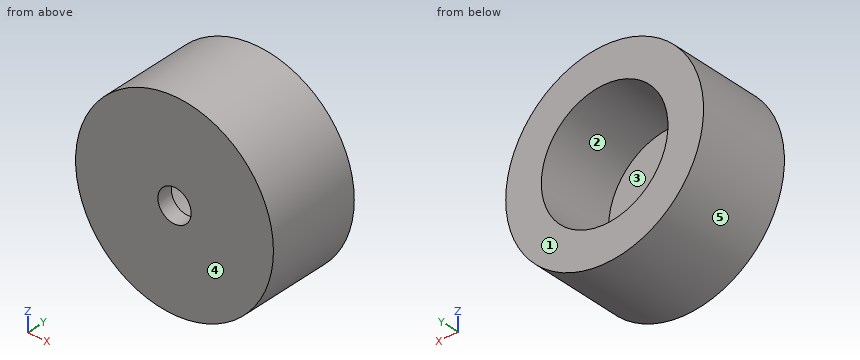
from build123d import *

# Parameters (mm, degrees)
SKETCH1_R           = 12.5
BOSS_EXTRUDE1_DEPTH = 2
SKETCH2_R           = 12.5
SKETCH2_R_2         = 8
BOSS_EXTRUDE2_DEPTH = 10
SKETCH3_R           = 2.1
CUT_EXTRUDE1_DEPTH  = 10


with BuildPart() as part:
    # Sketch1 → Boss-Extrude1 (new body)
    with BuildSketch(Plane(origin=(0, 0, 0), x_dir=(1, 0, 0), z_dir=(0, 1, 0))):
        Circle(SKETCH1_R)
    extrude(amount=BOSS_EXTRUDE1_DEPTH)

    # Sketch2 → Boss-Extrude2 (add)
    with BuildSketch(Plane(origin=(0, 2, 0), x_dir=(1, 0, 0), z_dir=(0, 1, 0))):
        Circle(SKETCH2_R)
        Circle(SKETCH2_R_2, mode=Mode.SUBTRACT)
    extrude(amount=BOSS_EXTRUDE2_DEPTH)

    # Sketch3 → Cut-Extrude1 (cut)
    with BuildSketch(Plane(origin=(0, 2, 0), x_dir=(1, 0, 0), z_dir=(0, 1, 0))):
        Circle(SKETCH3_R)
    extrude(amount=-CUT_EXTRUDE1_DEPTH, mode=Mode.SUBTRACT)


solid = part.part
Check sheet for the modelled part. Datum: model origin and axes. Units: mm. Face numbers are marked on the shaded views. A direction names the side the tool comes from. Give positions to 0.01 mm unless a question says otherwise; leave off trailing zeros. Order: outer loops, then holes, each group sorted by start corner. A loop starts at its lowest first (then second) coordinate and runs counter-clockwise, first axis right, second up. Notation, with made-up numbers: M 74.5,-39.5 L 96.5,-39.5 A35 ccw 96.5,-0.5 Z; hole C -3.75,-29.5 d2. An arc over 180 degrees is marked long. Answer as CSV lines item,"result". Start each with the question number.
Item 1: Cross-section at A-A on x = 0. Enter the section's corners in (y, z).
Item 2: Cross-section at D-D on x = 4.75. Enter the section's corners in (y, z), plus the area to 3 significant figures.
Item 3: Thickness scan on line 1 (Z direction, x = 0, y = 1.25); line 2 (X direction, y = 6.25, z = 0). Record the ranges inside material, lowest first. Write a range as [from, to].
Item 4: Tool access check on the marked faces 1 and 2. Record the directions out of +Z, -Z, +X, -X, +Y, -Y that give a thin tool (end or side, any length) a straight path to the whole face; none if there is none.
Item 5: Mould release check, pull along X, two halves, no side actions. Record for the marked faces 3, 4 and 5: +X half, -X half, draft (parallel to the pull), parting line (faces both ways), or undercut.
Item 6: Cross-section at B-B on z = 0. Enter the section's corners in (x, y), plus the area to 3 significant figures.
Item 7: Cross-section at C-C on y = 4. Enter the section's corners in (x, z), plus the area to 3 significant figures.
Item 8: Gauge pin test, flat ends, axial feed: P1, Ø1, axis at y = 7.5, z = 9, coming from the +X side; P2, Ø10, axis at x = 1, z = -3.5, coming from the -Y side; P3, Ø1.5, axis at x = 5.5, z = 1, coming from the +Y side. Record the tip position at first contact, or that the pin passes through.
Established:
1,outline,"M 0,-12.5 L 12,-12.5 L 12,-8 L 2,-8 L 2,-2.1 L 0,-2.1 Z; M 0,2.1 L 2,2.1 L 2,8 L 12,8 L 12,12.5 L 0,12.5 Z"
2,outline,"M 0,-11.56 L 12,-11.56 L 12,-6.44 L 2,-6.44 L 2,6.44 L 12,6.44 L 12,11.56 L 0,11.56 Z"
2,area,"149 mm^2"
3,line 1,"z = [-12.5, -2.1], [2.1, 12.5]"
3,line 2,"x = [-12.5, -8], [8, 12.5]"
4,face 1,"+Z, -Z, +X, -X, +Y"
4,face 2,"+Y"
5,face 3,"undercut"
5,face 4,"draft"
5,face 5,"parting line"
6,outline,"M -12.5,0 L -2.1,0 L -2.1,2 L -8,2 L -8,12 L -12.5,12 Z; M 2.1,0 L 12.5,0 L 12.5,12 L 8,12 L 8,2 L 2.1,2 Z"
6,area,"132 mm^2"
7,outline,"C 0,0 d25; hole C 0,0 d16"
7,area,"290 mm^2"
8,P1,"stops at x = 9.17"
8,P2,"stops at y = 0"
8,P3,"stops at y = 2"
